Can you work these out from the model? Positions are in its coordinate system, mm. Coordinates: 2 decimals unless noted, no trailing zeros. Order: outer loops, then holes, each group sorted by start corner. A loop starts at its lowest first (then second) coordinate and runs counter-clockwise, first axis right, second up. Notation, with made-up numbers: (2, 37.5) -> (19, 37.5) arc R34 cw to (19, 68.5) -> close; hole circle Ø6 at (74, 68.25). An arc over 180 degrees is marked (long way). Use a Markdown table: item, result. Add a question column.
1. Suppose I cut it at A-A, the plane y = 13. List the corners of the cut face in (x, z) for me, then the cut area to 3 significant figures.
2. If I drill on line 1 along X through (y, z) = (2.5, -2) (3 decimals); line 2 along Y through (x, z) = (-42, -5.65); line 3 along X through (y, z) = (11.5, -2), over which ranges is the centre line in solid material (lowest first)? Write a range as from..to.
3. Suppose I cut it at B-B, the plane x = 28. List the corners of the cut face in (y, z) for me.
4. For pin 1 Ø6.5 at (x, z) = (28.5, -1.5) entering from +Y; pin 2 Ø2.5 at (x, z) = (-27.175, -2) entering from -Y; pin 3 Ø3 at (x, z) = (-27, -1) entering from +Y, each with a flat end and sliding along its axis, tell me the tip position at first contact or that it passes through.
5. Suppose I cut it at C-C, the plane y = 2.75. List the corners of the cut face in (x, z) for me (3 decimals), then the cut area to 3 significant figures.
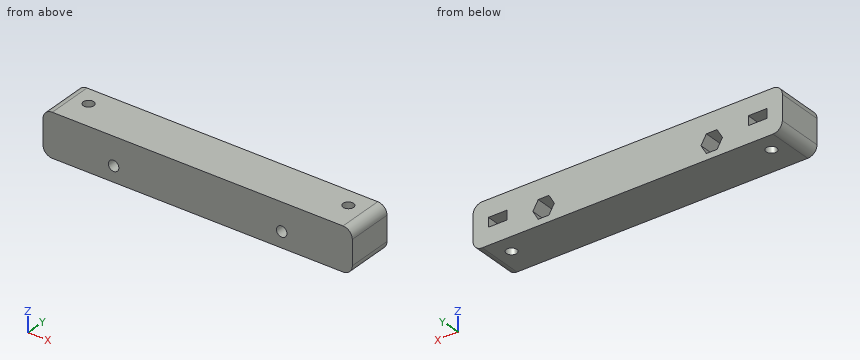
```python
from build123d import *

# Parameters (mm, degrees)
SKETCH1_W           = 100
SKETCH1_H           = 14
SKETCH1_R           = 1.7
BOSS_EXTRUDE1_DEPTH = 15
SKETCH3_R           = 1.7
CUT_EXTRUDE2_DEPTH  = 55.046276467
CUT_EXTRUDE3_START  = -7
CUT_EXTRUDE3_DEPTH  = 1.5
CUT_EXTRUDE4_DEPTH  = 6
FILLET4_R           = 3


with BuildPart() as part:
    # Sketch1 → Boss-Extrude1 (new body)
    with BuildSketch(Plane(origin=(0, 0, 0), x_dir=(1, 0, 0), z_dir=(0, 1, 0))):
        Rectangle(SKETCH1_W, SKETCH1_H)
        with Locations(Location((-27.175, 2, 0), (0, 0, 270))):
            Circle(SKETCH1_R, mode=Mode.SUBTRACT)
        with Locations(Location((27.175, 2, 0), (0, 0, 270))):
            Circle(SKETCH1_R, mode=Mode.SUBTRACT)
    extrude(amount=BOSS_EXTRUDE1_DEPTH)

    # Sketch3 → Cut-Extrude2 (cut, through all)
    with BuildSketch(Plane.XY.offset(7)):
        with Locations((-42, 9)):
            Circle(SKETCH3_R)
        with Locations((42, 9)):
            Circle(SKETCH3_R)
    extrude(amount=-CUT_EXTRUDE2_DEPTH, mode=Mode.SUBTRACT)

    # Sketch4 → Cut-Extrude3 (cut, symmetric)
    with BuildSketch(Plane.XY.offset(7).offset(CUT_EXTRUDE3_START)):
        Polygon((-45, 10.732050808), (-45, 16.451909609), (-39, 16.451909609), (-39, 10.732050808), (-39, 7.267949192), (-42, 5.535898385), (-45, 7.267949192), align=None)
        Polygon((39, 16.451909609), (39, 10.732050808), (39, 7.267949192), (42, 5.535898385), (45, 7.267949192), (45, 10.732050808), (45, 16.451909609), align=None)
    extrude(amount=CUT_EXTRUDE3_DEPTH, both=True, mode=Mode.SUBTRACT)

    # Sketch5 → Cut-Extrude4 (cut)
    with BuildSketch(Plane(origin=(0, 15, 0), x_dir=(1, 0, 0), z_dir=(0, 1, 0))):
        Polygon((-23.710898385, 2), (-25.442949192, 5), (-28.907050808, 5), (-30.639101615, 2), (-28.907050808, -1), (-25.442949192, -1), align=None)
        Polygon((25.442949192, -1), (23.710898385, 2), (25.442949192, 5), (28.907050808, 5), (30.639101615, 2), (28.907050808, -1), align=None)
    extrude(amount=-CUT_EXTRUDE4_DEPTH, mode=Mode.SUBTRACT)

    # Fillet4
    fillet4_edges = [part.edges().sort_by_distance(p)[0] for p in [
        (50, 7.5, 7),
        (-50, 7.5, 7),
        (-50, 7.5, -7),
        (50, 7.5, -7),
    ]]
    fillet(fillet4_edges, radius=FILLET4_R)


solid = part.part
```
Worked out:
| question | item | result |
|---|---|---|
| 1 | outline | (-50, -4) arc R3 ccw to (-47, -7) -> (47, -7) arc R3 ccw to (50, -4) -> (50, 4) arc R3 ccw to (47, 7) -> (-47, 7) arc R3 ccw to (-50, 4) -> close; hole (-45, -1.5) -> (-39, -1.5) -> (-39, 1.5) -> (-45, 1.5) -> close; hole (-30.64, -2) -> (-28.91, -5) -> (-25.44, -5) -> (-23.71, -2) -> (-25.44, 1) -> (-28.91, 1) -> close; hole (23.71, -2) -> (25.44, -5) -> (28.91, -5) -> (30.64, -2) -> (28.91, 1) -> (25.44, 1) -> close; hole (39, -1.5) -> (45, -1.5) -> (45, 1.5) -> (39, 1.5) -> close |
| 1 | area | 1,290 mm² |
| 2 | line 1 | x = -50..-28.875, -25.475..25.475, 28.875..50 |
| 2 | line 2 | y = 0..7.3, 10.7..15 |
| 2 | line 3 | x = -50..-30.64, -23.71..23.71, 30.64..50 |
| 3 | outline | (0, -7) -> (15, -7) -> (15, -5) -> (9, -5) -> (9, -3.49) -> (0, -3.49) -> close; (0, -0.51) -> (9, -0.51) -> (9, 1) -> (15, 1) -> (15, 7) -> (0, 7) -> close |
| 4 | pin 1 | stops at y = 15 |
| 4 | pin 2 | passes through |
| 4 | pin 3 | stops at y = 9 |
| 5 | outline | (-50, -4) arc R3 ccw to (-47, -7) -> (47, -7) arc R3 ccw to (50, -4) -> (50, 4) arc R3 ccw to (47, 7) -> (-47, 7) arc R3 ccw to (-50, 4) -> close; hole circle Ø3.4 at (-27.175, -2); hole circle Ø3.4 at (27.175, -2) |
| 5 | area | 1,370 mm² |
